Design review of the part built by this model. Coordinates are the model's own, in mm. A direction names the side the tool comes from. Give positions to 0.01 mm unless a question says otherwise; leave off trailing zeros. Loops run counter-clockwise (first coordinate to the right, second up) from the corner with the lowest first, then second, coordinate; pieces in that order, holes last. Notation, with made-up numbers: (-6.75, -28.5) - (30.25, -28.5) arc R20 cw to (30.25, -17.5) - close; hole circle Ø8 at (29, 86.25). An arc over 180 degrees is marked (long way). Write each question's results on one line, items separated by ' | '.
from build123d import *

# Parameters (mm, degrees)
SKETCH1_R           = 25.34
BOSS_EXTRUDE1_DEPTH = 2
SKETCH2_W           = 5
SKETCH2_H           = 13
BOSS_EXTRUDE2_DEPTH = 4
SKETCH3_R           = 1.5
CUT_EXTRUDE1_DEPTH  = 3
SKETCH4_W           = 10
SKETCH4_H           = 5
SKETCH4_W_2         = 13
SKETCH4_H_2         = 8
CUT_EXTRUDE2_DEPTH  = 3
SKETCH7_R           = 25.34
SKETCH7_R_2         = 1.5
BOSS_EXTRUDE3_DEPTH = 4


with BuildPart() as part:
    # Sketch1 → Boss-Extrude1 (new body)
    with BuildSketch(Plane(origin=(0, 0, 0), x_dir=(1, 0, 0), z_dir=(0, 1, 0))):
        Circle(SKETCH1_R)
    extrude(amount=BOSS_EXTRUDE1_DEPTH)

    # Sketch2 → Boss-Extrude2 (add)
    with BuildSketch(Plane(origin=(0, 2, 0), x_dir=(1, 0, 0), z_dir=(0, 1, 0))):
        with Locations((14.73, 0)):
            Rectangle(SKETCH2_W, SKETCH2_H)
        with BuildLine():
            Line((22.416636679, 6.5), (19.7, 6.5))
            Line((19.7, 6.5), (19.7, -6.5))
            Line((19.7, -6.5), (22.416636679, -6.5))
            ThreePointArc((22.416636679, -6.5), (23.34, 0), (22.416636679, 6.5))
        make_face()
        with BuildLine():
            Line((-19.7, -6.5), (-22.416636679, -6.5))
            ThreePointArc((-22.416636679, -6.5), (-23.34, 0), (-22.416636679, 6.5))
            Line((-22.416636679, 6.5), (-19.7, 6.5))
            Line((-19.7, 6.5), (-19.7, -6.5))
        make_face()
        with Locations((-14.73, 0)):
            Rectangle(SKETCH2_W, SKETCH2_H)
    extrude(amount=BOSS_EXTRUDE2_DEPTH)

    # Sketch3 → Cut-Extrude1 (cut, through all)
    with BuildSketch(Plane(origin=(0, 2, 0), x_dir=(1, 0, 0), z_dir=(0, 1, 0))):
        with Locations((-15.421998898, 15.421998898)):
            Circle(SKETCH3_R)
        with Locations((15.421998898, -15.421998898)):
            Circle(SKETCH3_R)
    extrude(amount=-CUT_EXTRUDE1_DEPTH, mode=Mode.SUBTRACT)

    # Sketch4 → Cut-Extrude2 (cut, through all)
    with BuildSketch(Plane(origin=(0, 2, 0), x_dir=(1, 0, 0), z_dir=(0, 1, 0))):
        with Locations((0, 15)):
            Rectangle(SKETCH4_W, SKETCH4_H)
        with Locations((0, -15)):
            Rectangle(SKETCH4_W, SKETCH4_H)
        Rectangle(SKETCH4_W_2, SKETCH4_H_2)
    extrude(amount=-CUT_EXTRUDE2_DEPTH, mode=Mode.SUBTRACT)

    # Sketch7 → Boss-Extrude3 (add)
    with BuildSketch(Plane(origin=(0, 2, 0), x_dir=(1, 0, 0), z_dir=(0, 1, 0))):
        Circle(SKETCH7_R)
        with Locations((-15.421998898, 15.421998898)):
            Circle(SKETCH7_R_2, mode=Mode.SUBTRACT)
        with Locations((15.421998898, -15.421998898)):
            Circle(SKETCH7_R_2, mode=Mode.SUBTRACT)
        with BuildLine():
            ThreePointArc((18.280458496, -14.511389912), (13.300678554, -13.300678554), (14.511389912, -18.280458496))
            ThreePointArc((14.511389912, -18.280458496), (-16.503872273, -16.503872273), (-18.280458496, 14.511389912))
            ThreePointArc((-18.280458496, 14.511389912), (-13.300678554, 13.300678554), (-14.511389912, 18.280458496))
            ThreePointArc((-14.511389912, 18.280458496), (16.503872273, 16.503872273), (18.280458496, -14.511389912))
        make_face(mode=Mode.SUBTRACT)
    extrude(amount=BOSS_EXTRUDE3_DEPTH)


solid = part.part
(1) Draft analysis for pull direction Z (two halves, no side actions). For faces 4 (the flat face through (15, 6, 0)), 5 (the flat face through (19.7, 4, 0)), 6 (the cylindrical face through (23.408, 2.958, 9.705)), state which applies: pulls with the +Z half, pulls with the -Z half, needs draft (parallel to the pull), parting line crosses it, or undercut.
Answers below:
face 4: needs draft | face 5: undercut | face 6: parting line crosses it
(2) Tool access review of faces 1 (the flat face through (-15, 6, 0)), 2 (the flat face through (0, 1, -4)), 3 (the flat face through (17.23, 4, 0)): name each direction out of +Z, -Z, +X, -X, +Y, -Y from which nothing blocks a thin tool from reaching the whole face with its end or side.
Answers below:
face 1: +Z, -Z, +X, -X, +Y | face 2: +Y, -Y | face 3: +Y
(3) Take a section at C-C on y = 4.8. Give the boundary of the cut face in (x, z), plus the area to 3 significant figures.
Answers below:
outline: circle Ø50.68 at (0, 0); (-17.23, -6.5) - (-12.23, -6.5) - (-12.23, 6.5) - (-17.23, 6.5) - close; (12.23, -6.5) - (17.23, -6.5) - (17.23, 6.5) - (12.23, 6.5) - close; hole (-22.42, -6.5) arc R23.34 ccw to (-18.28, -14.51) arc R3 cw (long way) to (-14.51, -18.28) arc R23.34 ccw to (22.42, -6.5) - (19.7, -6.5) - (19.7, 6.5) - (22.42, 6.5) arc R23.34 ccw to (18.28, 14.51) arc R3 cw (long way) to (14.51, 18.28) arc R23.34 ccw to (-22.42, 6.5) - (-19.7, 6.5) - (-19.7, -6.5) - close; hole circle Ø3 at (-15.42, -15.42); hole circle Ø3 at (15.42, 15.42) | area: 554 mm2
(4) Wall thickness on line 1 along X through (y, z) = (4.85, -3.5); line 2 along Z through (x, y) = (21, 4.75); line 3 along X through (y, z) = (2.9, -2): over which ranges is each line inside the solid? List them lowest first. Write a range as from..to.
Answers below:
line 1: -25.1..-19.7, -17.23..-12.23, 12.23..17.23, 19.7..25.1 | line 2: -14.18..-10.19, -6.5..6.5, 10.19..14.18 | line 3: -25.26..-19.7, -17.23..-12.23, 12.23..17.23, 19.7..25.26
(5) Take a section at D-D on x = -16. Give the boundary of the cut face in (y, z).
Answers below:
outline: (0, -19.65) - (6, -19.65) - (6, -16.81) - (0, -16.81) - close; (0, -14.04) - (6, -14.04) - (6, -12.48) - (2, -12.48) - (2, -6.5) - (6, -6.5) - (6, 6.5) - (2, 6.5) - (2, 16.99) - (6, 16.99) - (6, 19.65) - (0, 19.65) - close
(6) Insertion check: P1, Ø2, axis at x = 15, y = 3.5, coming from the +Z side; P2, Ø1, axis at y = 0.5, z = -16, coming from the +X side; P3, Ø2, axis at x = 21.5, y = 3.5, coming from the -Z side; P4, Ø1.8, axis at x = 15.42, z = 15.42, coming from the -Y side. Each pin has a flat end and moves straight along its axis. Give the tip position at first contact, or say it passes through.
Answers below:
P1: z = 21.12 | P2: x = 20.05 | P3: z = -14.9 | P4: through
(7) Take a section at A-A on x = 0. Give the boundary of the cut face in (y, z).
Answers below:
outline: (0, -25.34) - (6, -25.34) - (6, -23.34) - (2, -23.34) - (2, -17.5) - (0, -17.5) - close; (0, -12.5) - (2, -12.5) - (2, -4) - (0, -4) - close; (0, 4) - (2, 4) - (2, 12.5) - (0, 12.5) - close; (0, 17.5) - (2, 17.5) - (2, 23.34) - (6, 23.34) - (6, 25.34) - (0, 25.34) - close
(8) Take a section at B-B on z = 0. Give the boundary of the cut face in (x, y).
Answers below:
outline: (-25.34, 0) - (-6.5, 0) - (-6.5, 2) - (-12.23, 2) - (-12.23, 6) - (-17.23, 6) - (-17.23, 2) - (-19.7, 2) - (-19.7, 6) - (-25.34, 6) - close; (6.5, 0) - (25.34, 0) - (25.34, 6) - (19.7, 6) - (19.7, 2) - (17.23, 2) - (17.23, 6) - (12.23, 6) - (12.23, 2) - (6.5, 2) - close
